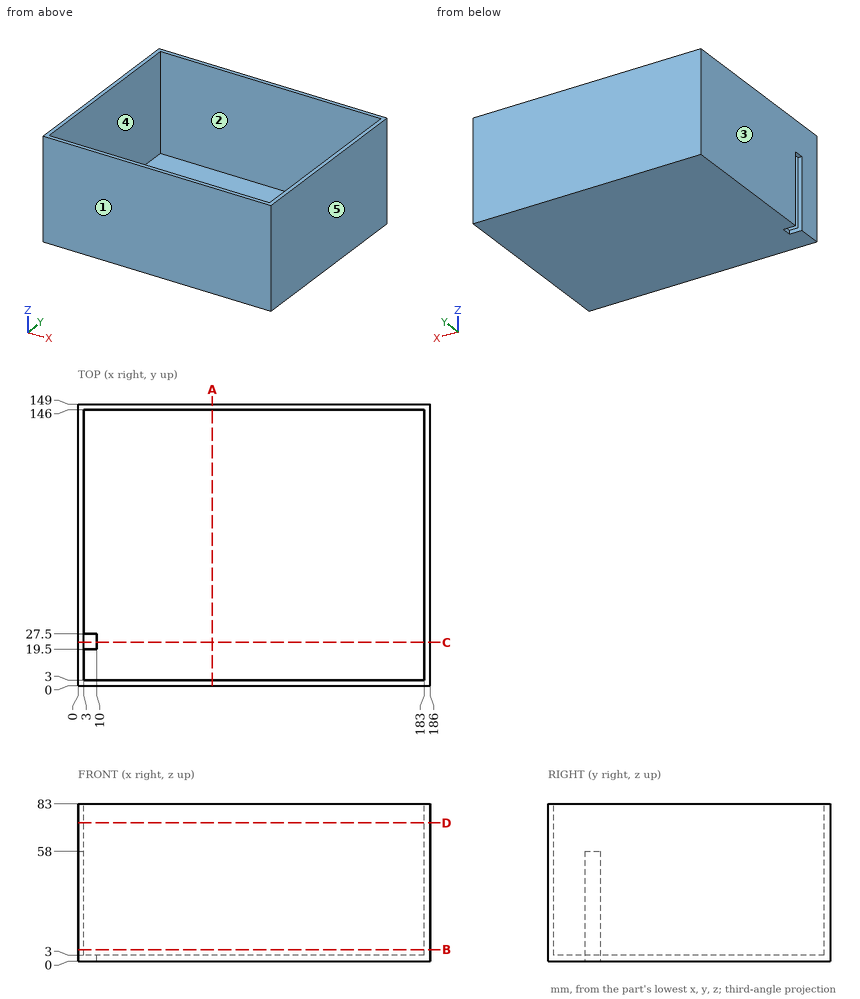
Drawing for the job (mm, zero at the part's lowest x, y, z). A direction names the side the tool comes from. Give positions to 0.01 mm unless a question says otherwise; leave off trailing zeros. Order: outer loops, then holes, each group sorted by start corner. A loop starts at its lowest first (then second) coordinate and runs counter-clockwise, first axis right, second up. Notation, with made-up numbers: M 74,2.5 L 94,2.5 A21 cw 94,29.5 Z; hole C -14.75,-8.75 d7. An arc over 180 degrees is marked long. Put each result on its own line as item: value. Start each with the question number.
(1) Saw through at B-B, the plane z = 6. Write the cut outline in (x, y), then the cut area to 3 significant figures.
(2) Saw through at A-A, the plane x = 71. Write the cut outline in (y, z).
(3) Saw through at C-C, the plane y = 23. Write the cut outline in (x, z).
(4) Drill centre lines: line 1 along X through (y, z) = (70, 26.5); line 2 along Y through (x, z) = (162, 23.5); line 3 along Z through (x, y) = (130, 26.5). Where is each one in solid material? Low to high.
(5) Mould opens along X. For the marked faces 1, 2 and 3 say: +X half, -X half, draft (parallel to the pull), parting line (faces both ways), or undercut.
(6) Which spindle directions (+Z, -Z, +X, -X, +Y, -Y) get a long thin tool onto all of the face, cutting with end or side? Do the marked faces 4 and 5. Say none if no direction does.
(7) Saw through at D-D, the plane z = 73. Write the cut outline in (x, y), then the cut area to 3 significant figures.
(8) Flat gauge pins, fed straight in: pin 1 Ø2.5 at (y, z) = (24.5, 1.5) entering from -X; pin 2 Ø0.9 at (x, y) = (1, 22) entering from -Z; pin 3 Ø3 at (x, y) = (89.5, 74.5) entering from +Z. Where does each tip first touch, or does it go through?
Check result:
1. outline: M 0,0 L 186,0 L 186,149 L 0,149 L 0,27.5 L 3,27.5 L 3,146 L 183,146 L 183,3 L 3,3 L 3,19.5 L 0,19.5 Z
1. area: 1,950 mm2
2. outline: M 0,0 L 149,0 L 149,83 L 146,83 L 146,3 L 3,3 L 3,83 L 0,83 Z
3. outline: M 0,58 L 3,58 L 3,83 L 0,83 Z; M 10,0 L 186,0 L 186,83 L 183,83 L 183,3 L 10,3 Z
4. line 1: x = 0 to 3, 183 to 186
4. line 2: y = 0 to 3, 146 to 149
4. line 3: z = 0 to 3
5. face 1: draft
5. face 2: undercut
5. face 3: -X half
6. face 4: +Z
6. face 5: +Z, -Z, +X, +Y, -Y
7. outline: M 0,0 L 186,0 L 186,149 L 0,149 Z; hole M 3,3 L 183,3 L 183,146 L 3,146 Z
7. area: 1,970 mm2
8. pin 1: stops at x = 10
8. pin 2: stops at z = 58
8. pin 3: stops at z = 3
